```python
from build123d import *

# Parameters (mm, degrees)
SKETCH_1_R      = 9.5
SKETCH_1_W      = 13
SKETCH_1_H      = 3
EXTRUDE_1_DEPTH = 3
CHAMFER_1_SIZE  = 1


with BuildPart() as part:
    # 草图1 → 凸台-拉伸1 (new body)
    with BuildSketch(Plane(origin=(0, 0, 0), x_dir=(0, 0, -1), z_dir=(1, 0, 0))):
        with BuildLine():
            Line((13, 6.1), (-13, 6.1))
            Line((-13, 6.1), (-13, 2.01))
            ThreePointArc((-13, 2.01), (-12.289357685, 1.715642315), (-11.995, 1.005))
            ThreePointArc((-11.995, 1.005), (-12.289357685, 0.294357685), (-13, 0))
            Line((-13, 0), (-16.5, 0))
            Line((-16.5, 0), (-16.5, -8))
            Line((-16.5, -8), (-13, -8))
            ThreePointArc((-13, -8), (-12.289357685, -8.294357685), (-11.995, -9.005))
            ThreePointArc((-11.995, -9.005), (-12.289357685, -9.715642315), (-13, -10.01))
            Line((-13, -10.01), (-13, -16.173762079))
            ThreePointArc((-13, -16.173762079), (-7.16028893, -36.474831388), (11.314290923, -26.231514557))
            Line((11.314290923, -26.231514557), (13, -16.173762079))
            Line((13, -16.173762079), (13, -10.01))
            ThreePointArc((13, -10.01), (11.995, -9.005), (13, -8))
            Line((13, -8), (16.5, -8))
            Line((16.5, -8), (16.5, 0))
            Line((16.5, 0), (13, 0))
            ThreePointArc((13, 0), (11.995, 1.005), (13, 2.01))
            Line((13, 2.01), (13, 6.1))
        make_face()
        with Locations((-2, -24)):
            Circle(SKETCH_1_R, mode=Mode.SUBTRACT)
        with Locations((0, -8.6)):
            Rectangle(SKETCH_1_W, SKETCH_1_H, mode=Mode.SUBTRACT)
        with BuildLine():
            Line((5.59, -3.1), (-5.59, -3.1))
            ThreePointArc((-5.59, -3.1), (-6.595, -4.105), (-7.6, -3.1))
            Line((-7.6, -3.1), (-7.6, 1.09))
            ThreePointArc((-7.6, 1.09), (-8.605, 2.095), (-7.6, 3.1))
            Line((-7.6, 3.1), (7.6, 3.1))
            ThreePointArc((7.6, 3.1), (8.310642315, 2.805642315), (8.605, 2.095))
            ThreePointArc((8.605, 2.095), (8.310642315, 1.384357685), (7.6, 1.09))
            Line((7.6, 1.09), (7.6, -3.1))
            ThreePointArc((7.6, -3.1), (6.595, -4.105), (5.59, -3.1))
        make_face(mode=Mode.SUBTRACT)
    extrude(amount=EXTRUDE_1_DEPTH)

    # 倒角1
    chamfer_1_edges = [part.edges().sort_by_distance(p)[0] for p in [
        (1.5, 6.1, 13),
        (1.5, 6.1, -13),
    ]]
    chamfer(chamfer_1_edges, length=CHAMFER_1_SIZE)


solid = part.part
```
Part model, mm, in its own coordinate system. A direction names the side the tool comes from. Give positions to 0.01 mm unless a question says otherwise; leave off trailing zeros. Loops run counter-clockwise (first coordinate to the right, second up) from the corner with the lowest first, then second, coordinate; pieces in that order, holes last. Notation, with made-up numbers: M 9.5,-8 L 55.5,-8 A30 cw 55.5,29 Z; hole C 43.25,-8 d2. An arc over 180 degrees is marked long. Return JSON: item names as keys, results as strings.
1) Saw through at D-D, the plane x = 2. Count the separate pieces of the cut face and the enclosed holes in it, then the cut area to 3 significant figures.
Calculated:
{"separate pieces": "1", "enclosed holes": "3", "area": "703 mm2"}
2) 3-axis set-ups, long thin cutter, end or side, ignore diameter. For faces 5 (the face through (1, 4, 13)), 6 (the face through (1, 0, -15)), 7 (the face through (1, -8, -15)), 8 (the face through (1.479, -4.105, -6.617)): which of +Z, -Z, +X, -X, +Y, -Y reach the whole face in a straight line?
Calculated:
{"face 5": "+Z, +X, -X, +Y", "face 6": "-Z, +X, -X, +Y", "face 7": "-Z, +X, -X, -Y", "face 8": "+X, -X"}
3) Flat gauge pins, fed straight in: pin 1 Ø1.5 at (x, z) = (1.5, 0) entering from -Y; pin 2 Ø0.9 at (x, y) = (1.5, -12) entering from -Z; pin 3 Ø1.5 at (x, y) = (1, -9) entering from -Z. Where does each tip first touch, or does it go through?
Calculated:
{"pin 1": "stops at y = -37.44", "pin 2": "stops at z = -13", "pin 3": "stops at z = -12.34"}
4) Pull direction Y, two halves, no side cores. Call faces 1 (the face through (1, -9, 6.5)), 2 (the face through (1.5, 5.6, -12.5)), 3 (the face through (1, -13, -13)), 4 (the face through (1, -8, 15)): released by +Y, released by -Y, zero draft, split by the parting line, or undercut.
Calculated:
{"face 1": "undercut", "face 2": "released by +Y", "face 3": "zero draft", "face 4": "undercut"}
5) Saw through at C-C, the plane y = -17.5. List the corners of the cut face in (x, z), then the cut area to 3 significant figures.
Calculated:
{"outline": "M 0,-12.78 L 3,-12.78 L 3,-4.93 L 0,-4.93 Z; M 0,8.93 L 3,8.93 L 3,13.83 L 0,13.83 Z", "area": "38.3 mm2"}
6) Saw through at A-A, the plane z = 2. List the corners of the cut face in (x, y), then the cut area to 3 significant figures.
Calculated:
{"outline": "M 0,-37.5 L 3,-37.5 L 3,-33.5 L 0,-33.5 Z; M 0,-14.5 L 3,-14.5 L 3,-10.1 L 0,-10.1 Z; M 0,-7.1 L 3,-7.1 L 3,-3.1 L 0,-3.1 Z; M 0,3.1 L 3,3.1 L 3,6.1 L 0,6.1 Z", "area": "46.2 mm2"}
7) Saw through at B-B, the plane z = 11. List the corners of the cut face in (x, y).
Calculated:
{"outline": "M 0,-34.06 L 3,-34.06 L 3,-27.04 L 0,-27.04 Z; M 0,-20.96 L 3,-20.96 L 3,6.1 L 0,6.1 Z"}
8) Drill centre lines: line 1 (Y direction, x = 1.1, z = 2); line 2 (Y direction, x = 1.45, z = 6); line 3 (Y direction, x = 0.8, z = 7). Where is each one in solid material? Low to high.
Calculated:
{"line 1": "y = -37.5 to -33.5, -14.5 to -10.1, -7.1 to -3.1, 3.1 to 6.1", "line 2": "y = -36.89 to -32.62, -15.38 to -10.1, -7.1 to -3.91, 3.1 to 6.1", "line 3": "y = -36.54 to -32.08, -15.92 to -4.02, 3.1 to 6.1"}
